The listing builds one solid part. Answer for the finished solid, in the listing's coordinates (mm). A direction names the side the tool comes from. Give positions to 0.01 mm unless a question says otherwise; leave off trailing zeros. Write each loop counter-clockwise with the first axis right and the second up, starting at its lowest first coordinate (ties: lowest second). Pieces come first, ordered by that corner, then holes. Notation, with made-up numbers: (84, 86) -> (137, 86) arc R15 cw to (137, 103) -> close; hole circle Ø11 at (49.25, -11). An arc over 180 degrees is marked (long way). Use CSV: the item, a comma, the result in double quotes. Start each with the question number.
Autodesk Inventor part; units mm, degrees
ref_plane "Work Plane1" through (-75, -725, 15) normal (0, 0, -1) x (0, 1, 0)
ref_plane "YZ Plane" through (0, 0, 0) normal (1, 0, 0) x (0, 1, 0)
ref_plane "XZ Plane" through (0, 0, 0) normal (0, 1, 0) x (-1, 0, 0)
sketch "Sketch1" plane through (0, 0, 0) normal (0, 0, 1) x (1, 0, 0)
  circle A0 centre (5, 95) radius 3 construction
  arc A1 (-53, -30) -> (-47, -30) centre (-50, -30) ccw construction
  line L0 (-53, -30) -> (-53, 30) construction
  arc A2 (-47, 30) -> (-53, 30) centre (-50, 30) ccw construction
  line L1 (-47, 30) -> (-47, -30) construction
  arc A3 (47, -30) -> (53, -30) centre (50, -30) ccw construction
  line L2 (47, -30) -> (47, 30) construction
  arc A4 (53, 30) -> (47, 30) centre (50, 30) ccw construction
  line L3 (53, 30) -> (53, -30) construction
  circle A5 centre (31.5, 31.5) radius 6 construction
  circle A6 centre (-31.5, 31.5) radius 6 construction
  circle A7 centre (-31.5, -31.5) radius 6 construction
  circle A8 centre (31.5, -31.5) radius 6 construction
  line L4 (62.5, 47.5) -> (-62.5, 47.5) construction
  line L5 (-62.5, 47.5) -> (-62.5, -47.5) construction
  line L6 (-62.5, -47.5) -> (62.5, -47.5) construction
  line L7 (62.5, -47.5) -> (62.5, 47.5) construction
  line L8 (62.5, -47.5) -> (-62.5, -47.5)
  line L9 (-62.5, -47.5) -> (-62.5, 132.5)
  line L10 (-62.5, 132.5) -> (62.5, 132.5)
  line L11 (62.5, 132.5) -> (62.5, -47.5)
  point P0 (0, 0)
  dimension "d0" = 180
  dimension "d1" = 125
ref_plane "Work Plane1" through (-75, -725, 15) normal (0, 0, -1) x (0, 1, 0)
extrude "Extrusion1" add sketch "Sketch1" along normal up to surface (15 mm away)
sketch "Sketch2" plane through (0, 0, 0) normal (0, 0, -1) x (-1, 0, 0)
  line L0 (-62.5, -47.5) -> (62.5, -47.5)
  arc A0 (47, -30) -> (53, -30) centre (50, -30) ccw construction
  arc A1 (53, 30) -> (47, 30) centre (50, 30) ccw construction
  line L1 (47, 30) -> (47, -30) construction
  line L2 (53, -30) -> (53, 30) construction
  point P0 (0, 0)
  point P1 (50, -25)
  point P2 (50, 0)
  point P3 (50, 25)
  point P4 (-50, -25)
  point P5 (-50, 0)
  point P6 (-50, 25)
  point P7 (50, 50)
  point P8 (-50, 50)
  dimension "d5" = 55
  dimension "d8" = 25
  dimension "d11" = 100
hole "Hole1" at (-50, -25, 0) at (-50, 0, 0) at (-50, 25, 0) at (50, -25, 0) at (50, 0, 0) at (50, 25, 0) at (-50, 50, 0) at (50, 50, 0) direction (0, 0, 1) diameter 4.917 end through all
sketch "Sketch4" plane through (0, 0, 0) normal (0, 0, -1) x (-1, 0, 0)
  circle A0 centre (-5, 95) radius 3
  line L0 (0, -83.5) -> (0, 168.5)
  line L1 (-10, 95) -> (10, 95) construction
  line L2 (-10, 92) -> (10, 92)
  line L3 (-10, 98) -> (10, 98)
  arc A1 (10, 92) -> (10, 98) centre (10, 95) ccw
  arc A2 (-10, 98) -> (-10, 92) centre (-10, 95) ccw
  line L4 (-62.5, 47.5) -> (62.5, 47.5) construction
  line L5 (-10, 26.134) -> (10, 26.134) construction
  line L6 (-10, 23.134) -> (10, 23.134)
  line L7 (-10, 29.134) -> (10, 29.134)
  arc A3 (10, 23.134) -> (10, 29.134) centre (10, 26.134) ccw
  arc A4 (-10, 29.134) -> (-10, 23.134) centre (-10, 26.134) ccw
  point P0 (0, 0)
  dimension "d21" = 20
  dimension "d22" = 3
  dimension "d23" = 3
  dimension "d24" = 6
  dimension "d27" = 47.5
  dimension "d30" = 68.866
extrude "Extrusion2" cut sketch "Sketch4" against normal blind 15
sketch "Sketch5" plane through (0, 0, 0) normal (0, 0, -1) x (-1, 0, 0)
  arc A0 (10, 92) -> (10, 98) centre (10, 95) ccw
  line L0 (10, 92) -> (-10, 92)
  arc A1 (-10, 98) -> (-10, 92) centre (-10, 95) ccw
  line L1 (-10, 98) -> (10, 98)
  arc A2 (10, 23.134) -> (10, 29.134) centre (10, 26.134) ccw
  line L2 (10, 23.134) -> (-10, 23.134)
  arc A3 (-10, 29.134) -> (-10, 23.134) centre (-10, 26.134) ccw
  line L3 (-10, 29.134) -> (10, 29.134)
  arc A4 (10, 92) -> (10, 98) centre (10, 95) ccw
  line L4 (10, 92) -> (-10, 92)
  arc A5 (-10, 98) -> (-10, 92) centre (-10, 95) ccw
  line L5 (-10, 98) -> (10, 98)
  circle A6 centre (-50, 50) radius 2.4585
  circle A7 centre (50, 50) radius 2.4585
  circle A8 centre (-50, 25) radius 2.4585
  circle A9 centre (-50, 0) radius 2.4585
  circle A10 centre (-50, -25) radius 2.4585
  circle A11 centre (50, 25) radius 2.4585
  circle A12 centre (50, 0) radius 2.4585
  circle A13 centre (50, -25) radius 2.4585
  line L6 (-62.5, -47.5) -> (62.5, -47.5)
  line L7 (62.5, -47.5) -> (62.5, 132.5)
  line L8 (62.5, 132.5) -> (-62.5, 132.5)
  line L9 (-62.5, 132.5) -> (-62.5, -47.5)
  line L10 (-10, 89) -> (10, 89)
  line L11 (-10, 101) -> (10, 101)
  arc A14 (10, 89) -> (10, 101) centre (10, 95) ccw
  arc A15 (-10, 101) -> (-10, 89) centre (-10, 95) ccw
  line L12 (0, -83.5) -> (0, 168.5)
  line L13 (-10, 20.134) -> (10, 20.134)
  line L14 (-10, 32.134) -> (10, 32.134)
  arc A16 (10, 20.134) -> (10, 32.134) centre (10, 26.134) ccw
  arc A17 (-10, 32.134) -> (-10, 20.134) centre (-10, 26.134) ccw
  point P0 (0, 0)
  dimension "d35" = 12
  dimension "d36" = 6
  dimension "d37" = 6
  dimension "d38" = 6
  dimension "d41" = 68.866
extrude "Extrusion3" cut sketch "Sketch5" against normal blind 7 contours A0 L1 L12 L11 A14 L10 L0 | L12 L10 A15 L11 L1 A1 L0 | L14 A16 L13 L12 L2 A2 L3 | L12 L3 A3 L2 L13 A17 L14
properties part number "MacroBasePlate_V1"
Q1. Section C-C on z = 4.75 is taken. State how many separate pieces and enclosed holes the cut face has, then the cut area to 3 significant figures.
Q2. Section D-D on y = 25 is taken. Give the vertices of the cut face in (x, z).
Q3. Section B-B on y = 50 is taken. Give the vertices of the cut face in (x, z).
Q4. Section A-A on x = -50 is taken. Give the vertices of the cut face in (y, z), then the cut area to 3 significant figures.
Q5. The mould has two halves that part along X. Classify faces 1 (the face through (-1, 44, 15)), 2 (the face through (13, 95, 11)), 3 (the face through (-62.5, 41, 7)): +X half, -X half, draft (parallel to the pull), parting line (faces both ways), or undercut.
Q6. Straight lines are drawn through the part: L1, parallel to Y at x = 2, z = 5.25; L2, parallel to Y at x = 50, z = 11; L3, parallel to X at y = 25, z = 6.5. For each, find the intervals that lie inside material, in ascending order.
Q7. For faces 4 (the face through (1, -47.5, 7)), 5 (the face through (0, 29.134, 11)), 6 (the face through (0, 101, 3)), determine the directions among +Z, -Z, +X, -X, +Y, -Y from which every point of the face is accessible in a straight line to the end or side of a thin tool.
Output:
1,separate pieces,"1"
1,enclosed holes,"10"
1,area,"21,600 mm²"
2,outline,"(-62.5, 0) -> (-52.46, 0) -> (-52.46, 15) -> (-62.5, 15) -> close; (-47.54, 0) -> (-15.89, 0) -> (-15.89, 7) -> (-12.78, 7) -> (-12.78, 15) -> (-47.54, 15) -> close; (12.78, 7) -> (15.89, 7) -> (15.89, 0) -> (47.54, 0) -> (47.54, 15) -> (12.78, 15) -> close; (52.46, 0) -> (62.5, 0) -> (62.5, 15) -> (52.46, 15) -> close"
3,outline,"(-62.5, 0) -> (-52.46, 0) -> (-52.46, 15) -> (-62.5, 15) -> close; (-47.54, 0) -> (47.54, 0) -> (47.54, 15) -> (-47.54, 15) -> close; (52.46, 0) -> (62.5, 0) -> (62.5, 15) -> (52.46, 15) -> close"
4,outline,"(-47.5, 0) -> (-27.46, 0) -> (-27.46, 15) -> (-47.5, 15) -> close; (-22.54, 0) -> (-2.46, 0) -> (-2.46, 15) -> (-22.54, 15) -> close; (2.46, 0) -> (22.54, 0) -> (22.54, 15) -> (2.46, 15) -> close; (27.46, 0) -> (47.54, 0) -> (47.54, 15) -> (27.46, 15) -> close; (52.46, 0) -> (132.5, 0) -> (132.5, 15) -> (52.46, 15) -> close"
4,area,"2,400 mm²"
5,face 1,"draft"
5,face 2,"undercut"
5,face 3,"-X half"
6,L1,"-47.5 to 20.13, 32.13 to 89, 101 to 132.5"
6,L2,"-47.5 to -27.46, -22.54 to -2.46, 2.46 to 22.54, 27.46 to 47.54, 52.46 to 132.5"
6,L3,"-62.5 to -52.46, -47.54 to -15.89, 15.89 to 47.54, 52.46 to 62.5"
7,face 4,"+Z, -Z, +X, -X, -Y"
7,face 5,"+Z, -Z"
7,face 6,"-Z"
